from build123d import *

# Parameters (mm, degrees)
SKETCH007_W             = 425
SKETCH007_H             = 370
SKETCH007_W_2           = 379
SKETCH007_H_2           = 303
PAD003_DEPTH            = 20
PAD004_DEPTH            = 5
LINEARPATTERN001_COUNT  = 6
LINEARPATTERN001_PITCH  = 60
BODY001_ROLL_ANGLE      = 0.707143
BODY001_PITCH_ANGLE     = 0.707089
BODY001_PLACEMENT_ANGLE = 0.004364


with BuildPart() as part:
    # Sketch007 → Pad003 (new body)
    with BuildSketch(Plane.XY):
        Rectangle(SKETCH007_W, SKETCH007_H)
        with Locations((0, 10.5)):
            Rectangle(SKETCH007_W_2, SKETCH007_H_2, mode=Mode.SUBTRACT)
    extrude(amount=PAD003_DEPTH)

    # Sketch008 → Pad004 (join)
    with BuildSketch(Plane.XY):
        with BuildLine():
            ThreePointArc((-155.799344, -161.125363), (-159.299344, -164.625363), (-155.799344, -168.125363))
            Line((-155.799344, -168.125363), (-145.799344, -168.125363))
            ThreePointArc((-145.799344, -168.125363), (-142.299344, -164.625363), (-145.799344, -161.125363))
            Line((-155.799344, -161.125363), (-145.799344, -161.125363))
        make_face()
    pad004 = extrude(amount=-PAD004_DEPTH)

    # LinearPattern001: Pad004 ×6
    with Locations(*[(i * LINEARPATTERN001_PITCH, 0, 0) for i in range(1, LINEARPATTERN001_COUNT)]):
        add(pad004)


with BuildPart() as part_1:
    # Body001 roll: moved
    add(part.part.rotate(Axis((0, 0, 0), (1, 0, 0)), BODY001_ROLL_ANGLE))


with BuildPart() as part_2:
    # Body001 pitch: moved
    add(part_1.part.rotate(Axis((0, 0, 0), (0, 1, 0)), BODY001_PITCH_ANGLE))


with BuildPart() as part_3:
    # Body001 placement: moved
    add(part_2.part.moved(Location((-350, 290, 140))).rotate(Axis((-350, 290, 140), (0, 0, 1)), BODY001_PLACEMENT_ANGLE))


solid = part_3.part
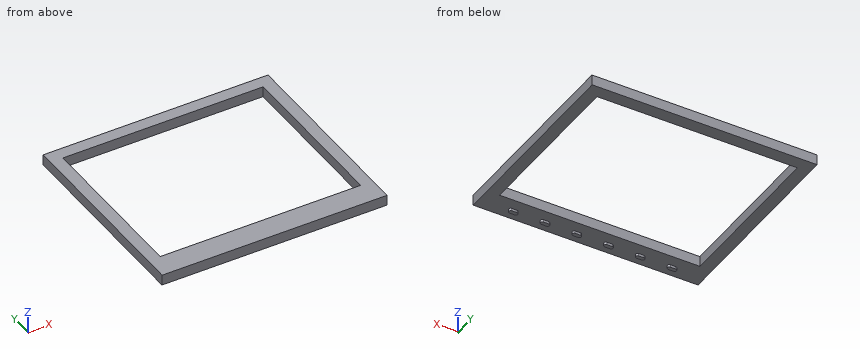
Geometry check sheet. Reference: the model listing, model coordinates, mm. Round coordinates to 2 decimals unless told otherwise and drop trailing zeros. Order: outer loops, then holes, each group sorted by start corner. A loop starts at its lowest first (then second) coordinate and runs counter-clockwise, first axis right, second up. Notation, with made-up numbers: M 31,-31.5 L 83,-31.5 A28 cw 83,-0.5 Z; hole C 28,41.25 d11. An arc over 180 degrees is marked long. Answer in a Markdown table with one row per item.
(1) Sectioned sample at B-B, the plane y = 223. Record the cut outline in (x, z), and give its area (3 significant figures).
Responses:
| item | result |
|---|---|
| outline | M -562.49,141.8 L -539.49,141.51 L -539.24,161.51 L -562.24,161.8 Z; M -160.52,136.83 L -137.52,136.55 L -137.27,156.55 L -160.27,156.83 Z |
| area | 920 mm² |
(2) Go/stop test with flat-tipped pins: P1, Ø12, axis at y = 244.5, z = 147.5, coming from the +X side; P2, Ø1, axis at y = 190.5, z = 140, coming from the +X side; P3, Ø1, axis at y = 224, z = 135.5, coming from the +X side; P4, Ø2, axis at x = -365, z = 138, coming from the -Y side. Record where each tip stops, or that it passes through.
Responses:
| item | result |
|---|---|
| P1 | stops at x = -137.31 |
| P2 | stops at x = -137.47 |
| P3 | passes through |
| P4 | stops at y = 105 |
(3) Sectioned sample at A-A, the plane x = -260.5. Record the cut outline in (y, z), and give its area (3 significant figures).
Responses:
| item | result |
|---|---|
| outline | M 104.77,156.61 L 105.02,136.61 L 121.89,136.82 L 121.96,131.82 L 128.96,131.91 L 128.89,136.91 L 149.02,137.16 L 148.77,157.16 Z; M 451.75,160.89 L 451.99,140.89 L 474.99,141.18 L 474.75,161.18 Z |
| area | 1,380 mm² |
(4) Scan lines: probe 1 along Y at (x, z) = (-474, 157); probe 2 along Y at (x, z) = (-212.5, 150.5); probe 3 along X at (y, z) = (230, 156). Record each from-to range of solid material in increasing order. Write a range as from..to.
Responses:
| item | result |
|---|---|
| probe 1 | y = 104.79..148.79, 451.81..474.81 |
| probe 2 | y = 104.85..148.85, 451.87..474.87 |
| probe 3 | x = -562.31..-539.31, -160.28..-137.28 |
